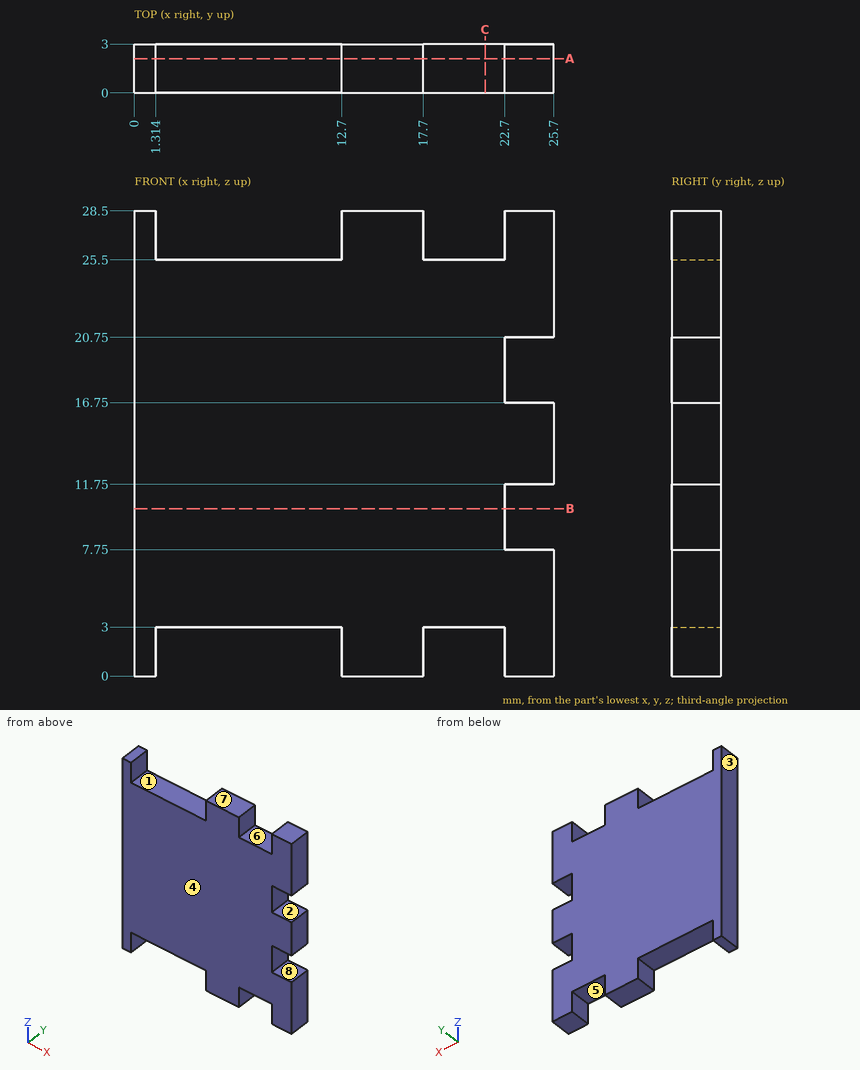
The figure shows three views and two pictorial views of one solid part (mm, origin at its lowest corner). Answer the questions. A direction names the side the tool comes from. Give positions to 0.01 mm unless a question says otherwise; leave off trailing zeros. Order: outer loops, then holes, each group sorted by start corner. A loop starts at its lowest first (then second) coordinate and runs counter-clockwise, first axis right, second up. Notation, with made-up numbers: M -16.75,88 L 10.25,88 A16 cw 10.25,102 Z; hole C -1,1 d6. An arc over 180 degrees is marked long. Return JSON: item names as keys, results as strings.
Q1. Which of the six approach directions +Z, -Z, +X, -X, +Y, -Y give full straight-line access (tool end or side, diameter ignored) to the marked faces 4, 5, 6, 7 and 8?
Answer below:
{"face 4": "+Z, -Z, +X, -X, -Y", "face 5": "-Z, +Y, -Y", "face 6": "+Z, +Y, -Y", "face 7": "+Z, +X, -X, +Y, -Y", "face 8": "+X, +Y, -Y"}
Q2. Each of these flat-tipped pins is pushed along its axis until it touches: pin 1 (0.9 mm diameter, centred on x = 6, y = 2, fed in from -Z); pin 2 (0.9 mm diameter, centred on x = 21.5, y = 1, fed in from +Z). Where does it stop, or does it pass through?
Answer below:
{"pin 1": "stops at z = 3", "pin 2": "stops at z = 25.5"}
Q3. The mould has two halves that part along Z. Classify the marked faces 1, 2 and 3: pulls with the +Z half, pulls with the -Z half, needs draft (parallel to the pull), parting line crosses it, or undercut.
Answer below:
{"face 1": "pulls with the +Z half", "face 2": "undercut", "face 3": "needs draft"}
Q4. Find section C-C, the plane x = 21.5. Write down the section's boundary in (y, z), and give its area (3 significant figures).
Answer below:
{"outline": "M 0,3 L 3,3 L 3,25.5 L 0,25.5 Z", "area": "67.5 mm^2"}
Q5. Find the intervals of material crossed by line 1 along X through (y, z) = (2.85, 27); line 2 along Z through (x, y) = (9.75, 2.75); line 3 along X through (y, z) = (1.85, 8.25), in increasing order. Write a range as [from, to].
Answer below:
{"line 1": "x = [0, 1.31], [12.7, 17.7], [22.7, 25.7]", "line 2": "z = [3, 25.5]", "line 3": "x = [0, 22.7]"}
Q6. Find section B-B, the plane z = 10.25. Write down the section's boundary in (x, y).
Answer below:
{"outline": "M 0,0 L 22.7,0 L 22.7,3 L 0,3 Z"}
Q7. Find section A-A, the plane y = 2.1. Write down the section's boundary in (x, z), and give its area (3 significant figures).
Answer below:
{"outline": "M 0,0 L 1.31,0 L 1.31,3 L 12.7,3 L 12.7,0 L 17.7,0 L 17.7,3 L 22.7,3 L 22.7,0 L 25.7,0 L 25.7,7.75 L 22.7,7.75 L 22.7,11.75 L 25.7,11.75 L 25.7,16.75 L 22.7,16.75 L 22.7,20.75 L 25.7,20.75 L 25.7,28.5 L 22.7,28.5 L 22.7,25.5 L 17.7,25.5 L 17.7,28.5 L 12.7,28.5 L 12.7,25.5 L 1.31,25.5 L 1.31,28.5 L 0,28.5 Z", "area": "610 mm^2"}
